from build123d import *

# Parameters (mm, degrees)
ESQUISSE1_R        = 40
BOSS_EXTRU_1_DEPTH = 10
CONG_1_R           = 10
ESQUISSE2_R        = 4
BOSS_EXTRU_2_DEPTH = 50


with BuildPart() as part:
    # Esquisse1 → Boss.-Extru.1 (new body)
    with BuildSketch(Plane.XY):
        Circle(ESQUISSE1_R)
    extrude(amount=BOSS_EXTRU_1_DEPTH)

    # Congé1
    cong_1_edges = [part.edges().sort_by_distance(p)[0] for p in [
        (-40, 0, 10),
    ]]
    fillet(cong_1_edges, radius=CONG_1_R - 0.0001)  # a hair under: the kernel refuses the full size

    # Esquisse2 → Boss.-Extru.2 (add)
    with BuildSketch(Plane.XY.offset(10)):
        Circle(ESQUISSE2_R)
    extrude(amount=BOSS_EXTRU_2_DEPTH)


solid = part.part
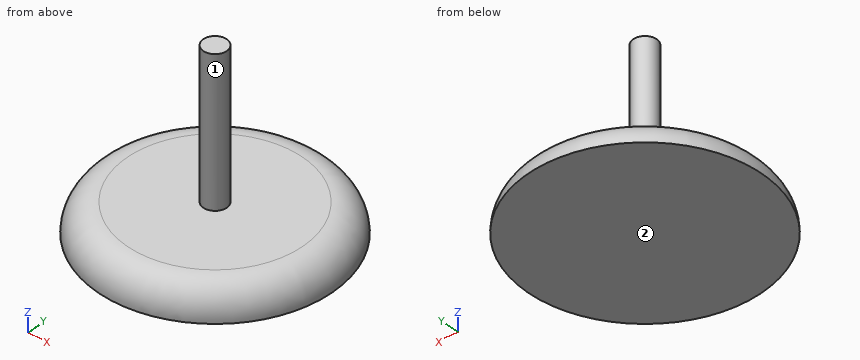
Geometry check sheet. Reference: the model listing, model coordinates, mm. Face numbers are marked on the shaded views. A direction names the side the tool comes from. Round coordinates to 2 decimals unless told otherwise and drop trailing zeros. Loops run counter-clockwise (first coordinate to the right, second up) from the corner with the lowest first, then second, coordinate; pieces in that order, holes last. Notation, with made-up numbers: (81, 71) -> (109, 71) arc R20 cw to (109, 76) -> close; hole circle Ø11 at (65.25, 25). An arc over 180 degrees is marked (long way). Answer as a JSON object with one key per item and string values. Group by question number.
Item 1: Depth check by flat-ended pin: pin 1 Ø1.5 at (x, y) = (5, -18.5) entering from +Z. Enter the tip coordinate at first touch or a pass-through.
Item 2: Set-up check for the marked faces 1 and 2: record each of +Z, -Z, +X, -X, +Y, -Y from which the full face is reachable in a straight line by a thin tool's end or side.
Item 3: Cross-section at D-D, the plane z = 6.5. Record the cut outline in (x, y).
Item 4: Thickness scan on line 1 along Z through (x, y) = (24, 16.5); line 2 along X through (y, z) = (1.5, 53.5); line 3 along Y through (x, z) = (3, 24). Record the ranges inside material, lowest first.
Item 5: Cross-section at C-C, the plane z = 19.5. Record the cut outline in (x, y).
Determined:
{
 "1": {"pin 1": "stops at z = 10"},
 "2": {"face 1": "+Z", "face 2": "-Z, +X, -X, +Y, -Y"},
 "3": {"outline": "circle Ø75.2 at (0, 0)"},
 "4": {"line 1": "z = 0 to 10", "line 2": "x = -3.71 to 3.71", "line 3": "y = -2.65 to 2.65"},
 "5": {"outline": "circle Ø8 at (0, 0)"}
}
